Here's how the part is built. I have some questions about the finished solid (model axes, mm). Face numbers are marked on the shaded views. Round coordinates to 2 decimals unless told otherwise and drop trailing zeros. Loops run counter-clockwise (first coordinate to the right, second up) from the corner with the lowest first, then second, coordinate; pieces in that order, holes last. Notation, with made-up numbers: (-32, 35) - (-27, 35) arc R16 ccw to (-27, 65) - close; hole circle Ø11 at (55.5, -30.5). An arc over 180 degrees is marked (long way). Answer as a JSON object with one key per item and string values. Group by question number.
1) If I drill on line 1 along Y through (x, z) = (-24.75, -1.8); line 2 along X through (y, z) = (9, -2.75); line 3 along X through (y, z) = (1.5, -2.25), over which ranges is the centre line in solid material (lowest first)? Write a range as [from, to].
2) I want a section at D-D, the plane z = -0.5. Please give me the cut outline in (x, y).
3) If we mould it in two halves opening along X, with no side actions, what happens to the marked faces 1, 2, 3 and 4? For each: pulls with the +X half, pulls with the -X half, needs draft (parallel to the pull), parting line crosses it, or undercut.
4) I want a section at B-B, the plane z = 3.25. Please give me the cut outline in (x, y).
5) I want a section at A-A, the plane x = -24.75. Please give me the cut outline in (y, z), then the cut area to 3 significant figures.
6) Will these pins go through, and if not, where does the flat tip stop? P1, Ø8, axis at x = -28, y = -3, coming from the +Z side; P2, Ø2.5, axis at y = -8.5, z = 2.5, coming from the +X side; P3, Ø11.5, axis at x = 24.75, y = 0, coming from the +Z side; P4, Ø3, axis at y = -10.5, z = -1.5, coming from the -X side.
7) I want a section at C-C, the plane y = 0. Please give me the cut outline in (x, z), then the cut area to 3 significant figures.
from build123d import *

# Parameters (mm, degrees)
F0_W     = 80
F0_H     = 30
F1_DEPTH = 4
F3_DEPTH = 3
F4_R     = 5
F4_R_2   = 1.7
F5_DEPTH = 5.001
F6_R     = 10


with BuildPart() as f1:
    # F0 (on Top) → F1 (new body, symmetric)
    with BuildSketch(Plane.XY):
        Rectangle(F0_W, F0_H)
    extrude(amount=F1_DEPTH, both=True)

    # F2 (on face) → F3 (cut)
    with BuildSketch(Plane.XY.offset(4)):
        with BuildLine():
            Line((-18.75, 15), (-30.75, 15))
            Line((-30.75, 15), (-30.75, 7.605669))
            Line((-30.75, 7.605669), (-30.75, -15))
            Line((-30.75, -15), (-18.75, -15))
            Line((-18.75, -15), (-18.75, -6))
            Line((-18.75, -6), (-12.123867, -6))
            ThreePointArc((-12.123867, -6), (-6.123867, 0), (-12.123867, 6))
            Line((-12.123867, 6), (-18.75, 6))
            Line((-18.75, 6), (-18.75, 15))
        make_face()
        with BuildLine():
            Line((30.75, -15), (30.75, 15))
            Line((30.75, 15), (18.75, 15))
            Line((18.75, 15), (18.75, 6))
            Line((18.75, 6), (12.123867, 6))
            ThreePointArc((12.123867, 6), (6.123867, 0), (12.123867, -6))
            Line((12.123867, -6), (18.75, -6))
            Line((18.75, -6), (18.75, -15))
            Line((18.75, -15), (30.75, -15))
        make_face()
    extrude(amount=-F3_DEPTH, mode=Mode.SUBTRACT)

    # F4 (on face) → F5 (cut, through all)
    with BuildSketch(Plane.XY.offset(1)):
        with Locations((-24.75, 0)):
            Circle(F4_R)
        with Locations((-24.75, 10)):
            Circle(F4_R_2)
        with Locations((-24.75, -10)):
            Circle(F4_R_2)
        with Locations((24.75, 10)):
            Circle(F4_R_2)
        with Locations((24.75, 0)):
            Circle(F4_R)
        with Locations((24.75, -10)):
            Circle(F4_R_2)
    extrude(amount=-F5_DEPTH, mode=Mode.SUBTRACT)

    # F6
    f6_edges = [f1.edges().sort_by_distance(p)[0] for p in [
        (-40, 15, 0),
        (-40, -15, 0),
        (40, 15, 0),
        (40, -15, 0),
    ]]
    fillet(f6_edges, radius=F6_R)


solid = f1.part
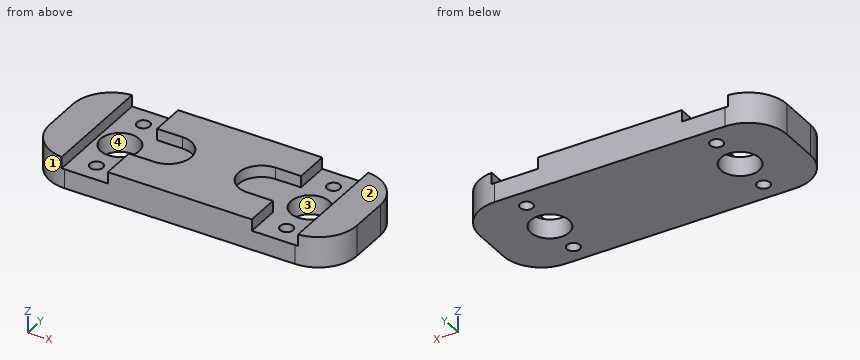
Outcome:
{
 "1": {"line 1": "[-15, -11.7], [-8.3, -5], [5, 8.3], [11.7, 15]", "line 2": "[-39.17, -26.12], [-23.38, 23.38], [26.12, 39.17]", "line 3": "[-40, -29.52], [-19.98, 19.98], [29.52, 40]"},
 "2": {"outline": "(-40, -5) arc R10 ccw to (-30, -15) - (30, -15) arc R10 ccw to (40, -5) - (40, 5) arc R10 ccw to (30, 15) - (-30, 15) arc R10 ccw to (-40, 5) - close; hole circle Ø10 at (-24.75, 0); hole circle Ø3.4 at (-24.75, -10); hole circle Ø3.4 at (-24.75, 10); hole circle Ø10 at (24.75, 0); hole circle Ø3.4 at (24.75, -10); hole circle Ø3.4 at (24.75, 10)"},
 "3": {"face 1": "pulls with the -X half", "face 2": "needs draft", "face 3": "undercut", "face 4": "undercut"},
 "4": {"outline": "(-40, -5) arc R10 ccw to (-30.75, -14.97) - (-30.75, 14.97) arc R10 ccw to (-40, 5) - close; (-18.75, -15) - (18.75, -15) - (18.75, -6) - (12.12, -6) arc R6 cw to (12.12, 6) - (18.75, 6) - (18.75, 15) - (-18.75, 15) - (-18.75, 6) - (-12.12, 6) arc R6 cw to (-12.12, -6) - (-18.75, -6) - close; (30.75, -14.97) arc R10 ccw to (40, -5) - (40, 5) arc R10 ccw to (30.75, 14.97) - close"},
 "5": {"outline": "(-15, -4) - (-11.7, -4) - (-11.7, 1) - (-15, 1) - close; (-8.3, -4) - (-5, -4) - (-5, 1) - (-8.3, 1) - close; (5, -4) - (8.3, -4) - (8.3, 1) - (5, 1) - close; (11.7, -4) - (15, -4) - (15, 1) - (11.7, 1) - close", "area": "66.0 mm^2"},
 "6": {"P1": "z = 4", "P2": "x = 39.74", "P3": "z = 1", "P4": "x = -39.17"},
 "7": {"outline": "(-40, -4) - (-29.75, -4) - (-29.75, 1) - (-30.75, 1) - (-30.75, 4) - (-40, 4) - close; (-19.75, -4) - (19.75, -4) - (19.75, 1) - (6.12, 1) - (6.12, 4) - (-6.12, 4) - (-6.12, 1) - (-19.75, 1) - close; (29.75, -4) - (40, -4) - (40, 4) - (30.75, 4) - (30.75, 1) - (29.75, 1) - close", "area": "392 mm^2"}
}
